Part model, mm, in its own coordinate system. A direction names the side the tool comes from. Coordinates: 2 decimals unless noted, no trailing zeros. Loops run counter-clockwise (first coordinate to the right, second up) from the corner with the lowest first, then second, coordinate; pieces in that order, holes last. Notation, with made-up numbers: M 49,-23.75 L 101,-23.75 A28 ccw 101,15.25 Z; hole C 41.5,72.5 d6. An arc over 180 degrees is marked long. Answer as a JSON object with one key per item and string values. Group by question number.
1. Saw through at B-B on z = 0. Write the cut outline in (x, y), then the cut area to 3 significant figures.
2. Saw through at A-A on x = 0. Write the cut outline in (y, z), then the cut area to 3 significant figures.
3. Drop flat-ended pins along their axis: pin 1 Ø2 at (y, z) = (13.5, -26.5) entering from +X; pin 2 Ø5 at (x, z) = (-78.5, -1.5) entering from -Y; pin 3 Ø5 at (y, z) = (36, 0) entering from +X. Give the stop position or say it passes through.
4. 3-axis set-ups, long thin cutter, end or side, ignore diameter. For faces 1 (the face through (-61.9, 0, 20.4)), 2 (the face through (-81, 7, 0)), 3 (the face through (-25, 39, 0)): which of +Z, -Z, +X, -X, +Y, -Y reach the whole face in a straight line?
5. Saw through at D-D on z = -39. Write the cut outline in (x, y), then the cut area to 3 significant figures.
6. Drill centre lines: L1, parallel to Z at x = -67, y = 63.5; L2, parallel to Y at x = 36, z = -51.5; L3, parallel to Y at x = 55.5, z = -40. Where is each one in solid material? Low to high.
7. Saw through at C-C on y = 81. Write the cut outline in (x, z).
from build123d import *

# Parameters (mm, degrees)
SKETCH1_R           = 70
BOSS_EXTRUDE2_DEPTH = 15
SKETCH2_R           = 65
BOSS_EXTRUDE3_DEPTH = 3
BOSS_EXTRUDE4_DEPTH = 5


with BuildPart() as part:
    # Sketch1 → Boss-Extrude2 (new body)
    with BuildSketch(Plane(origin=(0, 0, 0), x_dir=(1, 0, 0), z_dir=(0, 1, 0))):
        with Locations(Location((0, 0, 0), (0, 0, 270))):
            Circle(SKETCH1_R)
    extrude(amount=BOSS_EXTRUDE2_DEPTH)

    # Sketch2 → Boss-Extrude3 (add)
    with BuildSketch(Plane.XZ):
        with Locations(Location((0, 0, 0), (0, 0, 270))):
            Circle(SKETCH2_R)
    extrude(amount=BOSS_EXTRUDE3_DEPTH)

    # Sketch3 → Boss-Extrude4 (add, symmetric)
    with BuildSketch(Plane.XY):
        with BuildLine():
            Line((-25, 62), (-25, 7))
            Line((-25, 7), (-92, 7))
            Line((-92, 7), (-109.156726544, 37.506503148))
            ThreePointArc((-109.156726544, 37.506503148), (-82.509371405, 102.772350464), (-25, 62))
        make_face()
    extrude(amount=BOSS_EXTRUDE4_DEPTH, both=True)


solid = part.part
Outcome:
{
 "1": {"outline": "M -109.16,37.51 L -92,7 L -70,7 L -70,0 L -65,0 L -65,-3 L 65,-3 L 65,0 L 70,0 L 70,15 L -25,15 L -25,62 A45 ccw long Z", "area": "9,560 mm²"},
 "2": {"outline": "M -3,-65 L 0,-65 L 0,-70 L 15,-70 L 15,70 L 0,70 L 0,65 L -3,65 Z", "area": "2,490 mm²"},
 "3": {"pin 1": "stops at x = 65.19", "pin 2": "stops at y = 7", "pin 3": "stops at x = -25"},
 "4": {"face 1": "-Y", "face 2": "+Z, -Z, -X, -Y", "face 3": "+Z, -Z, +X, +Y"},
 "5": {"outline": "M -58.13,0 L -52,0 L -52,-3 L 52,-3 L 52,0 L 58.13,0 L 58.13,15 L -58.13,15 Z", "area": "2,060 mm²"},
 "6": {"L1": "z = -5 to 5", "L2": "y = -3 to 15", "L3": "y = 0 to 15"},
 "7": {"outline": "M -109.5,-5 L -30.37,-5 L -30.37,5 L -109.5,5 Z"}
}
